Here's how the part is built. I have some questions about the finished solid (model axes, mm). A direction names the side the tool comes from. Round coordinates to 2 decimals unless told otherwise and drop trailing zeros. Order: outer loops, then holes, each group sorted by start corner. A loop starts at its lowest first (then second) coordinate and runs counter-clockwise, first axis right, second up. Notation, with made-up numbers: (-29.75, -13.75) -> (-11.75, -13.75) arc R8 ccw to (-11.75, -8.75) -> close; hole circle Ø8 at (-31, -5). An arc over 180 degrees is marked (long way). Answer in a Markdown table with one row per item.
```python
from build123d import *

# Parameters (mm, degrees)
CROQUIS1_R              = 1.27
CROQUIS1_R_2            = 0.57
SALIENTE_EXTRUIR1_DEPTH = 1.8
CROQUIS2_W              = 4.4
CROQUIS2_H              = 6
SALIENTE_EXTRUIR2_DEPTH = 3.24
CROQUIS3_W              = 2.24
CROQUIS3_H              = 5
CORTAR_EXTRUIR2_DEPTH   = 3.9
CORTAR_EXTRUIR3_START   = -24.6
CROQUIS3_3_W            = 2.24
CROQUIS3_3_H            = 5
CORTAR_EXTRUIR3_DEPTH   = 3.9


with BuildPart() as part:
    # Croquis1 → Saliente-Extruir1 (new body)
    with BuildSketch(Plane.XY):
        with BuildLine():
            Line((9.7, -8.89), (-9.7, -8.89))
            ThreePointArc((-9.7, -8.89), (-11.821320344, -8.011320344), (-12.7, -5.89))
            Line((-12.7, -5.89), (-12.7, 5.89))
            ThreePointArc((-12.7, 5.89), (-11.821320344, 8.011320344), (-9.7, 8.89))
            Line((-9.7, 8.89), (9.7, 8.89))
            ThreePointArc((9.7, 8.89), (11.821320344, 8.011320344), (12.7, 5.89))
            Line((12.7, 5.89), (12.7, -5.89))
            ThreePointArc((12.7, -5.89), (11.821320344, -8.011320344), (9.7, -8.89))
        make_face()
        with Locations((-9.7, 5.89)):
            Circle(CROQUIS1_R, mode=Mode.SUBTRACT)
        with Locations(Location((9.7, 5.89, 0), (0, 0, 180))):
            Circle(CROQUIS1_R, mode=Mode.SUBTRACT)
        with Locations((9.7, -5.89)):
            Circle(CROQUIS1_R, mode=Mode.SUBTRACT)
        with Locations(Location((-9.7, -5.89, 0), (0, 0, 180))):
            Circle(CROQUIS1_R, mode=Mode.SUBTRACT)
        with Locations((-7.62, -5.89)):
            Circle(CROQUIS1_R_2, mode=Mode.SUBTRACT)
        with Locations((-5.08, -5.89)):
            Circle(CROQUIS1_R_2, mode=Mode.SUBTRACT)
        with Locations((-2.54, -5.89)):
            Circle(CROQUIS1_R_2, mode=Mode.SUBTRACT)
        with Locations((0, -5.89)):
            Circle(CROQUIS1_R_2, mode=Mode.SUBTRACT)
        with Locations((2.54, -5.89)):
            Circle(CROQUIS1_R_2, mode=Mode.SUBTRACT)
        with Locations((5.08, -5.89)):
            Circle(CROQUIS1_R_2, mode=Mode.SUBTRACT)
        with Locations((7.62, -5.89)):
            Circle(CROQUIS1_R_2, mode=Mode.SUBTRACT)
    extrude(amount=SALIENTE_EXTRUIR1_DEPTH)

    # Croquis2 → Saliente-Extruir2 (add)
    with BuildSketch(Plane.XY.offset(1.8)):
        with Locations((-10.1, 0)):
            Rectangle(CROQUIS2_W, CROQUIS2_H)
        with Locations((10.1, 0)):
            Rectangle(CROQUIS2_W, CROQUIS2_H)
    extrude(amount=SALIENTE_EXTRUIR2_DEPTH)

    # Croquis3 → Cortar-Extruir2 (cut)
    with BuildSketch(Plane(origin=(12.3, 0, 0), x_dir=(0, 0, -1), z_dir=(1, 0, 0))):
        with Locations((-3.42, 0)):
            Rectangle(CROQUIS3_W, CROQUIS3_H)
    extrude(amount=-CORTAR_EXTRUIR2_DEPTH, mode=Mode.SUBTRACT)

    # Croquis3<3> → Cortar-Extruir3 (cut)
    with BuildSketch(Plane(origin=(12.3, 0, 0), x_dir=(0, 0, -1), z_dir=(1, 0, 0)).offset(CORTAR_EXTRUIR3_START)):
        with Locations((-3.42, 0)):
            Rectangle(CROQUIS3_3_W, CROQUIS3_3_H)
    extrude(amount=CORTAR_EXTRUIR3_DEPTH, mode=Mode.SUBTRACT)


solid = part.part
```
1. Suppose I cut it at C-C on z = 1.1. State how many separate pieces and enclosed holes the cut face has, then the cut area to 3 significant figures.
Numbers:
| item | result |
|---|---|
| separate pieces | 1 |
| enclosed holes | 11 |
| area | 416 mm2 |
2. Please list where these lines run through material, in increasing order: line 1 along Y through (x, z) = (-9.7, 1); line 2 along Y through (x, z) = (-9.75, 2.7); line 3 along X through (y, z) = (6.25, 0.9).
Numbers:
| item | result |
|---|---|
| line 1 | y = -8.89 to -7.16, -4.62 to 4.62, 7.16 to 8.89 |
| line 2 | y = -3 to -2.5, 2.5 to 3 |
| line 3 | x = -12.68 to -10.92, -8.48 to 8.48, 10.92 to 12.68 |
3. Suppose I cut it at B-B on x = 10.25. Write out the boundary of the cut face in (y, z), then the cut area to 3 significant figures.
Numbers:
| item | result |
|---|---|
| outline | (-8.84, 0) -> (-7.03, 0) -> (-7.03, 1.8) -> (-8.84, 1.8) -> close; (-4.75, 0) -> (4.75, 0) -> (4.75, 1.8) -> (3, 1.8) -> (3, 5.04) -> (-3, 5.04) -> (-3, 1.8) -> (-4.75, 1.8) -> close; (7.03, 0) -> (8.84, 0) -> (8.84, 1.8) -> (7.03, 1.8) -> close; hole (-2.5, 2.3) -> (2.5, 2.3) -> (2.5, 4.54) -> (-2.5, 4.54) -> close |
| area | 31.8 mm2 |
4. For faces 1 (the face through (-10, -2.5, 3)), 2 (the face through (10, 3, 3)), 3 (the face through (10, 0, 2.3)), 4 (the face through (-12.3, 0, 4.8)), which set-ups out of +Z, -Z, +X, -X, +Y, -Y let a thin tool reach every point of the face, with its end or its side?
Numbers:
| item | result |
|---|---|
| face 1 | -X |
| face 2 | +Z, +X, -X, +Y |
| face 3 | +X |
| face 4 | +Z, -X, +Y, -Y |
5. We'd pull the mould along X, two halves only. Please class faces 5 (the face through (-10, 0, 5.04)), 6 (the face through (7.2, -5.505, 0.887)), 7 (the face through (-11.84, 7.99, 0.89)): released by +X, released by -X, zero draft, split by the parting line, or undercut.
Numbers:
| item | result |
|---|---|
| face 5 | zero draft |
| face 6 | undercut |
| face 7 | released by -X |
6. Suppose I cut it at A-A on x = -7.62. Write out the boundary of the cut face in (y, z), then the cut area to 3 significant figures.
Numbers:
| item | result |
|---|---|
| outline | (-8.89, 0) -> (-6.46, 0) -> (-6.46, 1.8) -> (-8.89, 1.8) -> close; (-5.32, 0) -> (8.89, 0) -> (8.89, 1.8) -> (-5.32, 1.8) -> close |
| area | 30.0 mm2 |
7. Suppose I cut it at D-D on y = 4.25. Write out the boundary of the cut face in (x, z), then the cut area to 3 significant figures.
Numbers:
| item | result |
|---|---|
| outline | (-12.7, 0) -> (12.7, 0) -> (12.7, 1.8) -> (-12.7, 1.8) -> close |
| area | 45.7 mm2 |
8. For pin 1 Ø0.7 at (x, y) = (7.62, -5.89) entering from +Z; pin 2 Ø0.7 at (x, z) = (11, 3.5) entering from +Y; pin 3 Ø1.6 at (x, z) = (10, 3.5) entering from -Y; pin 4 Ø1 at (x, y) = (-5, 6) entering from +Z, each with a flat end and sliding along its axis, tell me the tip position at first contact or that it passes through.
Numbers:
| item | result |
|---|---|
| pin 1 | passes through |
| pin 2 | stops at y = 3 |
| pin 3 | stops at y = -3 |
| pin 4 | stops at z = 1.8 |
